Source: CAD feature listing. Evaluate the final solid. Frame: model axes, mm. A direction names the side the tool comes from. Give positions to 0.01 mm unless a question says otherwise; leave off trailing zeros. Loops run counter-clockwise (first coordinate to the right, second up) from the corner with the lowest first, then second, coordinate; pieces in that order, holes last. Notation, with made-up numbers: (77.25, -21.75) - (87.25, -21.75) arc R25 ccw to (87.25, -8.75) - close; hole circle Ø11 at (6, -33.5). An arc over 180 degrees is marked (long way). Put each result on its own line as item: value.
```python
from build123d import *

# Parameters (mm, degrees)
SKETCH2_R           = 1.6
SKETCH2_W           = 20
SKETCH2_H           = 4.65
BOSS_EXTRUDE1_DEPTH = 5


with BuildPart() as part:
    # Sketch2 → Boss-Extrude1 (new body)
    with BuildSketch(Plane(origin=(0, 0, 0), x_dir=(1, 0, 0), z_dir=(0, 1, 0))):
        with BuildLine():
            Line((10, 0), (40, 0))
            ThreePointArc((40, 0), (47.071067812, 2.928932188), (50, 10))
            Line((50, 10), (50, 20))
            ThreePointArc((50, 20), (47.071067812, 27.071067812), (40, 30))
            Line((40, 30), (10, 30))
            ThreePointArc((10, 30), (2.928932188, 27.071067812), (0, 20))
            Line((0, 20), (0, 10))
            ThreePointArc((0, 10), (2.928932188, 2.928932188), (10, 0))
        make_face()
        with Locations((9, 5)):
            Circle(SKETCH2_R, mode=Mode.SUBTRACT)
        with Locations((41, 5)):
            Circle(SKETCH2_R, mode=Mode.SUBTRACT)
        with Locations((9, 22.675)):
            Circle(SKETCH2_R, mode=Mode.SUBTRACT)
        with Locations((41, 22.675)):
            Circle(SKETCH2_R, mode=Mode.SUBTRACT)
        with Locations((25, 22.675)):
            Rectangle(SKETCH2_W, SKETCH2_H, mode=Mode.SUBTRACT)
    extrude(amount=BOSS_EXTRUDE1_DEPTH)


solid = part.part
```
1) Section query C-C, the plane x = 9.5. Output: boundary loops of the cut face in (y, z), plus the area to 3 significant figures.
Check result:
outline: (0, -29.99) - (5, -29.99) - (5, -24.19) - (0, -24.19) - close; (0, -21.16) - (5, -21.16) - (5, -6.52) - (0, -6.52) - close; (0, -3.48) - (5, -3.48) - (5, -0.01) - (0, -0.01) - close
area: 119 mm²
2) Section query B-B, the plane z = -6. Output: boundary loops of the cut face in (x, y), plus the area to 3 significant figures.
Check result:
outline: (0.83, 0) - (7.75, 0) - (7.75, 5) - (0.83, 5) - close; (10.25, 0) - (39.75, 0) - (39.75, 5) - (10.25, 5) - close; (42.25, 0) - (49.17, 0) - (49.17, 5) - (42.25, 5) - close
area: 217 mm²
3) Access query for faces 1 (the flat face through (50, 2, -15)), 2 (the flat face through (25, 2, -20.35)). Directions: +Z, -Z, +X, -X, +Y, -Y. A direction counts if a zero-diameter tool reaches every point of the face in a straight line with its end or side. Return the directions, or none.
Check result:
face 1: +Z, -Z, +X, +Y, -Y
face 2: +Y, -Y
4) Material intervals for line 1 along Z through (x, y) = (28.5, 0.6); line 2 along X through (y, z) = (2.3, -5); line 3 along X through (y, z) = (3.7, -24), sorted ascending. Write a range as [from, to].
Check result:
line 1: [-30, -25], [-20.35, 0]
line 2: [1.34, 7.4], [10.6, 39.4], [42.6, 48.66]
line 3: [0.83, 8.1], [9.9, 15], [35, 40.1], [41.9, 49.17]
5) Section query A-A, the plane x = 29. Output: boundary loops of the cut face in (y, z).
Check result:
outline: (0, -30) - (5, -30) - (5, -25) - (0, -25) - close; (0, -20.35) - (5, -20.35) - (5, 0) - (0, 0) - close
6) Section query D-D, the plane y = 1.1. Output: boundary loops of the cut face in (x, z) (3 decimals), plus the area to 3 significant figures.
Check result:
outline: (0, -20) arc R10 ccw to (10, -30) - (40, -30) arc R10 ccw to (50, -20) - (50, -10) arc R10 ccw to (40, 0) - (10, 0) arc R10 ccw to (0, -10) - close; hole circle Ø3.2 at (9, -22.675); hole circle Ø3.2 at (9, -5); hole (15, -25) - (35, -25) - (35, -20.35) - (15, -20.35) - close; hole circle Ø3.2 at (41, -22.675); hole circle Ø3.2 at (41, -5)
area: 1,290 mm²
7) Mould query, pull axis Z, two halves, no side actions, for faces 3 (the flat face through (15, 2, -23)), 4 (the flat face through (0, 2, -15)), 5 (the cylindrical face through (47.15, 2.46, -26.99)), 6 (the cylindrical face through (7.73, 2.46, -4.03)). Classes: pulls with the +Z half, pulls with the -Z half, needs draft (parallel to the pull), parting line crosses it, or undercut.
Check result:
face 3: undercut
face 4: needs draft
face 5: pulls with the -Z half
face 6: undercut
8) Pin query (flat end, axial travel): P1, Ø1.5, axis at x = 42, y = 1, coming from the -Z side; P2, Ø1.9, axis at x = 41, z = -22.675, coming from the +Y side; P3, Ø2.5, axis at y = 3.5, z = -22.5, coming from the +X side; P4, Ø2, axis at x = 6.5, y = 1.5, coming from the +Z side. Return the tip coordinate at first contact, or that it passes through.
Check result:
P1: z = -29.92
P2: through
P3: x = 49.92
P4: z = -0.32
